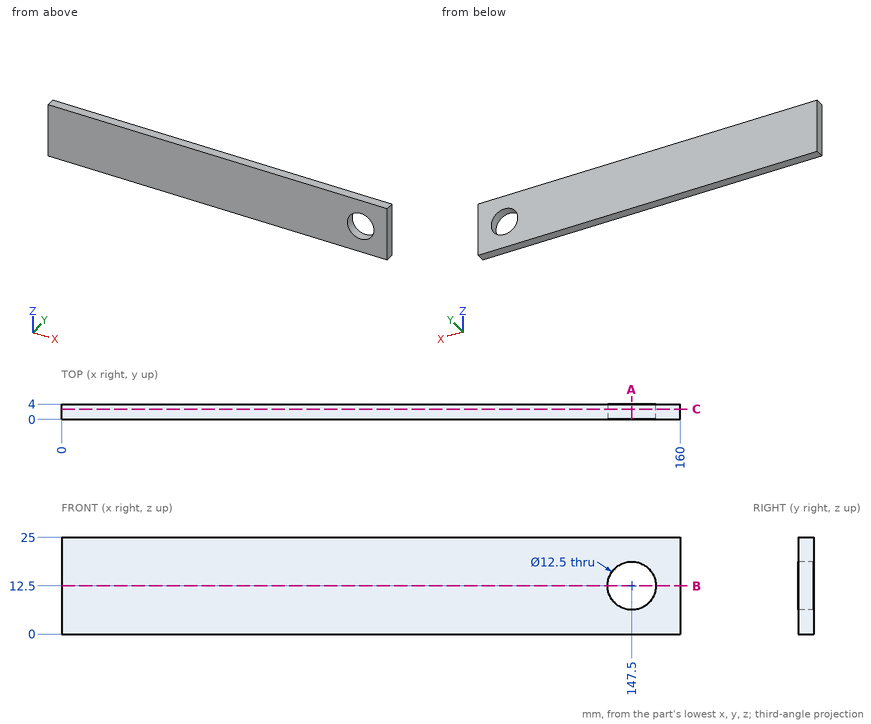
For this review, use the dimensioned drawing (mm, ordinates from the lowest corner) and the shaded views. Round coordinates to 2 decimals unless told otherwise and drop trailing zeros. Order: outer loops, then holes, each group sorted by start corner. A loop starts at its lowest first (then second) coordinate and runs counter-clockwise, first axis right, second up. Notation, with made-up numbers: M 6.25,19.5 L 59.25,19.5 A28 cw 59.25,39.5 Z; hole C 15.5,-23 d4. An arc over 180 degrees is marked long. Write each question's results on one line, items separated by ' | '. Start each with the question number.
1. Add section B-B (z = 12.5). State the section outline as (x, y) points, then the cut area to 3 significant figures.
2. Add section C-C (y = 2.7). State the section outline as (x, z) points.
3. Add section A-A (x = 147.5). State the section outline as (y, z) points.
4. To check wall thickness, follow L1, parallel to Z at x = 147.5, y = 2.6; L2, parallel to X at y = 2.25, z = 12.5. State the ranges of each line that lie inside material, in increasing order. Write a range as [from, to].
Output values:
1) outline: M 0,0 L 141.25,0 L 141.25,4 L 0,4 Z; M 153.75,0 L 160,0 L 160,4 L 153.75,4 Z | area: 590 mm^2
2) outline: M 0,0 L 160,0 L 160,25 L 0,25 Z; hole C 147.5,12.5 d12.5
3) outline: M 0,0 L 4,0 L 4,6.25 L 0,6.25 Z; M 0,18.75 L 4,18.75 L 4,25 L 0,25 Z
4) L1: [0, 6.25], [18.75, 25] | L2: [0, 141.25], [153.75, 160]
